Could you check a few things on this model? Use its own coordinates, in mm. Give positions to 0.01 mm unless a question says otherwise; leave off trailing zeros. Write each question's results on one line, items separated by ' | '. Start each with the question number.
from build123d import *

# Parameters (mm, degrees)
SKETCH1_R               = 1.6
BOSS_EXTRUDE1_DEPTH     = 6
CUT_EXTRUDE1_DEPTH      = 203.20197823
CUT_EXTRUDE1_DEPTH_BACK = 203.20197823
SKETCH4_R               = 1.6
CUT_EXTRUDE2_DEPTH      = 10
CUT_EXTRUDE3_DEPTH      = 10
FILLET1_R               = 5
SKETCH6_R               = 1.125
CUT_EXTRUDE4_DEPTH      = 10
SKETCH7_R               = 1.55
CUT_EXTRUDE5_DEPTH      = 10


with BuildPart() as part:
    # Sketch1 → Boss-Extrude1 (new body)
    with BuildSketch(Plane(origin=(0, 0, 0), x_dir=(1, 0, 0), z_dir=(0, 1, 0))):
        Polygon((-145, 120), (125, 120), (125, -100.8), (125, -140.8), (-145, -140.8), (-145, -100.8), align=None)
        with Locations(Location((-100, -5, 0), (0, 0, 270))):
            Circle(SKETCH1_R, mode=Mode.SUBTRACT)
        with Locations(Location((80, -5, 0), (0, 0, 270))):
            Circle(SKETCH1_R, mode=Mode.SUBTRACT)
        with Locations(Location((-55, -5, 0), (0, 0, 270))):
            Circle(SKETCH1_R, mode=Mode.SUBTRACT)
        with Locations(Location((35, -5, 0), (0, 0, 270))):
            Circle(SKETCH1_R, mode=Mode.SUBTRACT)
    extrude(amount=BOSS_EXTRUDE1_DEPTH)

    # Sketch3 → Cut-Extrude1 (cut, two sides: drawn at the far end of the back side and taken through both)
    with BuildSketch(Plane(origin=(0, 6, 0), x_dir=(1, 0, 0), z_dir=(0, 1, 0)).offset(-CUT_EXTRUDE1_DEPTH_BACK)):
        with BuildLine():
            Line((-28, 85), (-28, 120))
            Line((-28, 120), (28, 120))
            Line((28, 120), (28, 85))
            ThreePointArc((28, 85), (0, 57), (-28, 85))
        make_face()
    extrude(amount=CUT_EXTRUDE1_DEPTH + CUT_EXTRUDE1_DEPTH_BACK, mode=Mode.SUBTRACT)

    # Sketch4 → Cut-Extrude2 (cut)
    with BuildSketch(Plane.XZ):
        with Locations(Location((107, -110, 0), (0, 0, 270))):
            Circle(SKETCH4_R)
        with Locations(Location((-127, -110, 0), (0, 0, 270))):
            Circle(SKETCH4_R)
        with Locations(Location((107, 130.8, 0), (0, 0, 270))):
            Circle(SKETCH4_R)
        with Locations(Location((-127, 130.8, 0), (0, 0, 270))):
            Circle(SKETCH4_R)
    extrude(amount=-CUT_EXTRUDE2_DEPTH, mode=Mode.SUBTRACT)

    # Sketch5 → Cut-Extrude3 (cut)
    with BuildSketch(Plane(origin=(0, 6, 0), x_dir=(1, 0, 0), z_dir=(0, 1, 0))):
        with BuildLine():
            Line((-33.4, 110), (-33.4, 85))
            ThreePointArc((-33.4, 85), (-35, 83.4), (-36.6, 85))
            Line((-36.6, 85), (-36.6, 110))
            ThreePointArc((-36.6, 110), (-35, 111.6), (-33.4, 110))
        make_face()
        with BuildLine():
            Line((33.4, 110), (33.4, 85))
            ThreePointArc((33.4, 85), (35, 83.4), (36.6, 85))
            Line((36.6, 85), (36.6, 110))
            ThreePointArc((36.6, 110), (35, 111.6), (33.4, 110))
        make_face()
    extrude(amount=-CUT_EXTRUDE3_DEPTH, mode=Mode.SUBTRACT)

    # Fillet1
    fillet1_edges = [part.edges().sort_by_distance(p)[0] for p in [
        (-28, 3, -120),
        (28, 3, -120),
    ]]
    fillet(fillet1_edges, radius=FILLET1_R)

    # Sketch6 → Cut-Extrude4 (cut)
    with BuildSketch(Plane(origin=(0, 6, 0), x_dir=(1, 0, 0), z_dir=(0, 1, 0))):
        with Locations(Location((25.75, -55.149373751, 0), (0, 0, 270))):
            Circle(SKETCH6_R)
        with Locations(Location((-45.75, -55.149373751, 0), (0, 0, 270))):
            Circle(SKETCH6_R)
        with Locations(Location((-45.75, -126.649373751, 0), (0, 0, 270))):
            Circle(SKETCH6_R)
        with Locations(Location((25.75, -126.649373751, 0), (0, 0, 270))):
            Circle(SKETCH6_R)
        with BuildLine():
            Line((-40, -87.899373751), (20, -87.899373751))
            ThreePointArc((20, -87.899373751), (23, -90.899373751), (20, -93.899373751))
            Line((20, -93.899373751), (-40, -93.899373751))
            ThreePointArc((-40, -93.899373751), (-43, -90.899373751), (-40, -87.899373751))
        make_face()
        with BuildLine():
            Line((-40.316760433, -77.325947728), (20.316760433, -77.325947728))
            ThreePointArc((20.316760433, -77.325947728), (23.316760433, -80.325947728), (20.316760433, -83.325947728))
            Line((20.316760433, -83.325947728), (-40.316760433, -83.325947728))
            ThreePointArc((-40.316760433, -83.325947728), (-43.316760433, -80.325947728), (-40.316760433, -77.325947728))
        make_face()
        with BuildLine():
            Line((-40.436008981, -66.571059525), (20.436008981, -66.571059525))
            ThreePointArc((20.436008981, -66.571059525), (23.436008981, -69.571059525), (20.436008981, -72.571059525))
            Line((20.436008981, -72.571059525), (-40.436008981, -72.571059525))
            ThreePointArc((-40.436008981, -72.571059525), (-43.436008981, -69.571059525), (-40.436008981, -66.571059525))
        make_face()
        with BuildLine():
            Line((-30, -58.021465569), (10, -58.021465569))
            ThreePointArc((10, -58.021465569), (12.570860459, -60.592326028), (10, -63.163186487))
            Line((10, -63.163186487), (-30, -63.163186487))
            ThreePointArc((-30, -63.163186487), (-32.570860459, -60.592326028), (-30, -58.021465569))
        make_face()
        with BuildLine():
            Line((-30, -123.777281933), (10, -123.777281933))
            ThreePointArc((10, -123.777281933), (12.570860459, -121.206421475), (10, -118.635561016))
            Line((10, -118.635561016), (-30, -118.635561016))
            ThreePointArc((-30, -118.635561016), (-32.570860459, -121.206421475), (-30, -123.777281933))
        make_face()
        with BuildLine():
            Line((-40.436008981, -115.227687978), (20.436008981, -115.227687978))
            ThreePointArc((20.436008981, -115.227687978), (23.436008981, -112.227687978), (20.436008981, -109.227687978))
            Line((20.436008981, -109.227687978), (-40.436008981, -109.227687978))
            ThreePointArc((-40.436008981, -109.227687978), (-43.436008981, -112.227687978), (-40.436008981, -115.227687978))
        make_face()
        with BuildLine():
            Line((-40.316760433, -104.472799775), (20.316760433, -104.472799775))
            ThreePointArc((20.316760433, -104.472799775), (23.316760433, -101.472799775), (20.316760433, -98.472799775))
            Line((20.316760433, -98.472799775), (-40.316760433, -98.472799775))
            ThreePointArc((-40.316760433, -98.472799775), (-43.316760433, -101.472799775), (-40.316760433, -104.472799775))
        make_face()
    extrude(amount=-CUT_EXTRUDE4_DEPTH, mode=Mode.SUBTRACT)

    # Sketch7 → Cut-Extrude5 (cut)
    with BuildSketch(Plane(origin=(0, 6, 0), x_dir=(1, 0, 0), z_dir=(0, 1, 0))):
        with Locations(Location((-100, -27, 0), (0, 0, 270))):
            Circle(SKETCH7_R)
        with Locations(Location((-55, -27, 0), (0, 0, 270))):
            Circle(SKETCH7_R)
        with Locations(Location((35, -27, 0), (0, 0, 270))):
            Circle(SKETCH7_R)
        with Locations(Location((80, -27, 0), (0, 0, 270))):
            Circle(SKETCH7_R)
    extrude(amount=-CUT_EXTRUDE5_DEPTH, mode=Mode.SUBTRACT)


solid = part.part
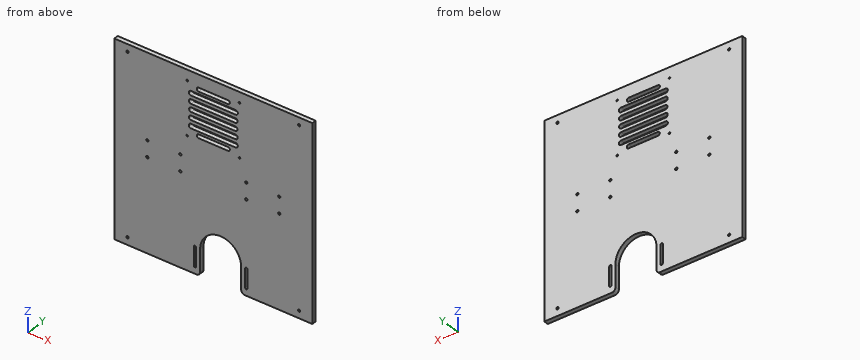
Q1. If we section it at A-A (y = 1.85): Count the separate pieces of the cut face and the enclosed holes in it, plus the area to 3 significant figures.
Q2. I'm going to push flat-ended pins straight in: P1, Ø1.5, axis at x = -26.5, z = -63.5, coming from the -Y side; P2, Ø1.5, axis at x = 13.5, y = 5.5, coming from the -Z side. Where does each tip first touch, or does it pass through?
Q3. Please list where these lines run through material, in increasing order: line 1 (X direction, y = 1.6, z = 5); line 2 (X direction, y = 1.95, z = -105); line 3 (X direction, y = 3.15, z = 27). Write a range as [from, to].
Determined:
1) separate pieces: 1 | enclosed holes: 25 | area: 64,500 mm²
2) P1: stops at y = 0 | P2: stops at z = -60.9
3) line 1: x = [-145, -101.6], [-98.4, -56.6], [-53.4, 33.4], [36.6, 78.4], [81.6, 125] | line 2: x = [-145, -36.6], [-33.4, -28], [28, 33.4], [36.6, 125] | line 3: x = [-145, -101.55], [-98.45, -56.55], [-53.45, 33.45], [36.55, 78.45], [81.55, 125]
